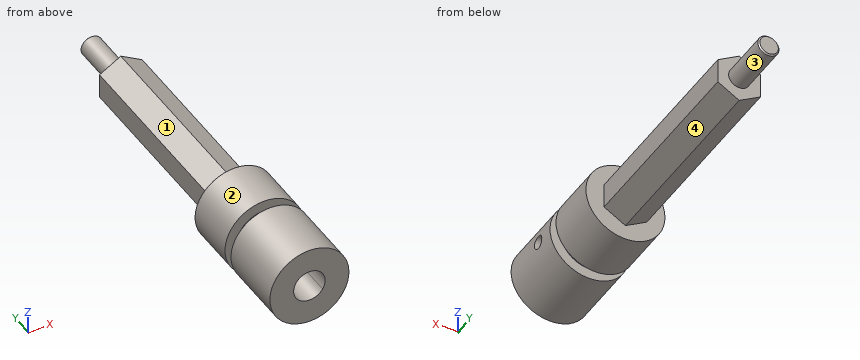
from build123d import *
from build123d.topology import SkipClean

# Parameters (mm, degrees)
SKETCH_1_R          = 7.5
EXTRUDE_1_DEPTH     = 25
EXTRUDE_2_DEPTH     = 38
CUT_EXTRUDE_1_DEPTH = 15
SKETCH_6_R          = 3
CUT_EXTRUDE_2_DEPTH = 3
M3X0_5_1_D          = 2.5
M3X0_5_1_DEPTH      = 5
SKETCH_21_R         = 3
CUT_EXTRUDE_3_DEPTH = 15
SKETCH_3_R          = 2
EXTRUDE_3_DEPTH     = 10
CHAMFER_1_SIZE      = 0.25
SKETCH_22_W         = 3.619891
SKETCH_22_H         = 2


with BuildPart() as part:
    # Sketch 1 → Extrude 1 (new body)
    with BuildSketch(Plane(origin=(0, 0, 0), x_dir=(1, 0, 0), z_dir=(0, 1, 0))):
        with Locations(Location((0, 0, 0), (0, 0, 270))):  # turned: the seam where the file's is
            Circle(SKETCH_1_R)
    extrude(amount=EXTRUDE_1_DEPTH)

    # Sketch 2 → Extrude 2 (add)
    with BuildSketch(Plane(origin=(0, 25, 0), x_dir=(1, 0, 0), z_dir=(0, 1, 0))):
        Polygon((0, -4.676537), (4.05, -2.338269), (4.05, 2.338269), (0, 4.676537), (-4.05, 2.338269), (-4.05, -2.338269), align=None)
    extrude(amount=EXTRUDE_2_DEPTH)

    # Sketch 5 → Cut-Extrude 1 (cut)
    with BuildSketch(Plane.XZ):
        with BuildLine():
            Line((2.5, 1.658312), (2.5, -1.658312))
            ThreePointArc((2.5, -1.658312), (-3, 0), (2.5, 1.658312))
        make_face()
    extrude(amount=-CUT_EXTRUDE_1_DEPTH, mode=Mode.SUBTRACT)

    # Sketch 6 → Cut-Extrude 2 (cut)
    with SkipClean():  # keep this step's faces unmerged: merging them makes the solid invalid here
        with BuildSketch(Plane.XZ):
            with Locations(Location((0, 0, 0), (0, 0, 270))):  # turned: the seam where the file's is
                Circle(SKETCH_6_R)
        extrude(amount=-CUT_EXTRUDE_2_DEPTH, mode=Mode.SUBTRACT)

    # M3x0.5 _1
    with Locations(Plane.ZY.offset(-2.5)):
        with Locations((0, 9)):
            Hole(M3X0_5_1_D / 2, depth=M3X0_5_1_DEPTH)

    # Sketch 21 → Cut-Extrude 3 (cut)
    with SkipClean():  # keep this step's faces unmerged: merging them makes the solid invalid here
        with BuildSketch(Plane.XZ):
            with Locations(Location((0, 0, 0), (0, 0, 270))):  # turned: the seam where the file's is
                Circle(SKETCH_21_R)
        extrude(amount=-CUT_EXTRUDE_3_DEPTH, mode=Mode.SUBTRACT)

    # Sketch 3 → Extrude 3 (add)
    with SkipClean():  # keep this step's faces unmerged: merging them makes the solid invalid here
        with BuildSketch(Plane(origin=(0, 63, 0), x_dir=(1, 0, 0), z_dir=(0, 1, 0))):
            with Locations(Location((0, 0, 0), (0, 0, 270))):  # turned: the seam where the file's is
                Circle(SKETCH_3_R)
        extrude(amount=EXTRUDE_3_DEPTH)

    # Chamfer 1
    chamfer_1_edges = [part.edges().sort_by_distance(p)[0] for p in [
        (0, 73, -2),
    ]]
    chamfer(chamfer_1_edges, length=CHAMFER_1_SIZE)

    # Sketch 22 → Cut-Revolve 1 (revolve, cut)
    with SkipClean():  # keep this step's faces unmerged: merging them makes the solid invalid here
        with BuildSketch(Plane.XY, mode=Mode.PRIVATE) as cut_revolve_1_sk:
            with Locations((7.309945, 14)):
                Rectangle(SKETCH_22_W, SKETCH_22_H)
        revolve(cut_revolve_1_sk.sketch.rotate(Axis((0, 25, 0), (0, -1, 0)), 90), axis=Axis((0, 25, 0), (0, -1, 0)), mode=Mode.SUBTRACT)  # turned: the seam where the file's is


solid = part.part
Here's how the part is built. I have some questions about the finished solid (model axes, mm). Face numbers are marked on the shaded views. A direction names the side the tool comes from. Round coordinates to 2 decimals unless told otherwise and drop trailing zeros. Loops run counter-clockwise (first coordinate to the right, second up) from the corner with the lowest first, then second, coordinate; pieces in that order, holes last. Notation, with made-up numbers: (-29.75, 31.5) - (-18.75, 31.5) arc R21 ccw to (-18.75, 63.5) - close; hole circle Ø2 at (-16.75, -10). An arc over 180 degrees is marked (long way). One line per question, with ' | ' between items. Start each with the question number.
Q1. Will these pins go through, and if not, where does the flat tip stop? pin 1 (5 mm diameter, centred on y = 36, z = -3, fed in from +X); pin 2 (6 mm diameter, centred on y = 45, z = 1, fed in from -X); pin 3 (3 mm diameter, centred on x = -6, y = 32.5, fed in from +Z); pin 4 (5 mm diameter, centred on x = -4.5, y = 8.5, fed in from +Z).
Q2. I want a section at C-C (y = 45). Write out the boundary of the cut face in (x, z).
Q3. For the marked faces 1, 2, 3 and 4, which set-ups out of +Z, -Z, +X, -X, +Y, -Y let a thin tool reach every point of the face, with its end or its side?
Q4. Please list where these lines run through material, in increasing order: line 1 (Y direction, x = 3.75, z = 5.5); line 2 (X direction, y = 4, z = 0); line 3 (Y direction, x = 4.65, z = 0). Write a range as [from, to].
Q5. I want a section at B-B (y = 14). Write out the boundary of the cut face in (x, z).
Q6. I want a section at D-D (z = 6.25). Write out the boundary of the cut face in (x, y), then the cut area to 3 significant figures.
Response values:
1) pin 1: stops at x = 4.05 | pin 2: stops at x = -4.05 | pin 3: passes through | pin 4: stops at z = 7.23
2) outline: (-4.05, -2.34) - (0, -4.68) - (4.05, -2.34) - (4.05, 2.34) - (0, 4.68) - (-4.05, 2.34) - close
3) face 1: +Z, -X, +Y | face 2: +Y, -Y | face 3: +Y | face 4: -Z, +X, +Y
4) line 1: y = [0, 13], [15, 25] | line 2: x = [-7.5, -3], [3, 7.5] | line 3: y = [0, 7.75], [10.25, 25]
5) outline: circle Ø11 at (0, 0); hole circle Ø6 at (0, 0)
6) outline: (-4.15, 0) - (4.15, 0) - (4.15, 13) - (-4.15, 13) - close; (-4.15, 15) - (4.15, 15) - (4.15, 25) - (-4.15, 25) - close | area: 191 mm²
